Geometry check sheet. Reference: the model listing, model coordinates, mm. A direction names the side the tool comes from. Round coordinates to 2 decimals unless told otherwise and drop trailing zeros. Loops run counter-clockwise (first coordinate to the right, second up) from the corner with the lowest first, then second, coordinate; pieces in that order, holes last. Notation, with made-up numbers: (-29.5, 83.25) -> (-13.5, 83.25) arc R21 cw to (-13.5, 108.25) -> close; hole circle Ø4 at (75, -26). An arc over 180 degrees is marked (long way). Use a Markdown table: item, result. Add a question column.
Q1. Gauge pin test, flat ends, axial feed: P1, Ø5, axis at x = 7.5, z = 0, coming from the -Y side; P2, Ø1, axis at x = -1.5, z = 0, coming from the +Y side; P3, Ø2, axis at x = 7.5, z = 2, coming from the -Y side. Record the tip position at first contact, or that the pin passes through.
Q2. Set-up check for faces 4 (the face through (17.27, -0.9, 2.86)), 5 (the face through (22.152, 2, -1)), 6 (the face through (12.902, 3, 1)): record each of +Z, -Z, +X, -X, +Y, -Y from which the full face is reachable in a straight line by a thin tool's end or side.
Q3. Release check for a two-part mould opening along X. For faces 1 (the face through (16.21, -0.98, 3.11)), 2 (the face through (5, -3, 0)), 3 (the face through (-5.56, -0.71, -2.04)) record: released by +X, released by -X, zero draft, split by the parting line, or undercut.
Q4. Material ranges on L1, parallel to Y at x = 2.25, z = 0; L2, parallel to Z at x = 20.5, y = 1; L3, parallel to Z at x = 9, y = 0.75, recorded low to high.
Q5. Sectioned sample at A-A, the plane z = 0. Enter the section's corners in (x, y), then the cut area to 4 significant figures.
Q6. Sectioned sample at C-C, the plane x = 12.5. Enter the section's corners in (y, z), then the cut area to 3 significant figures.
Q7. Sectioned sample at B-B, the plane y = 0. Enter the section's corners in (x, z).
```python
from build123d import *

# Parameters (mm, degrees)
CUT_EXTRUDE1_DEPTH      = 10
CUT_EXTRUDE1_DEPTH_BACK = 10


with BuildPart() as part:
    # Sketch1 → Revolve1 (revolve)
    with BuildSketch(Plane.XY, mode=Mode.PRIVATE) as revolve1_sk:
        Polygon((22.151518872, 3), (17.651518872, 4.5), (17.651518872, 3), (16.901518872, 3), (12.901518872, 4.5), (12.901518872, 3), (-7.848481128, 3), (-7.848481128, 2), (22.151518872, 2), align=None)
    revolve(revolve1_sk.sketch.rotate(Axis((0, 0, 0), (1, 0, 0)), 90), axis=Axis((0, 0, 0), (1, 0, 0)))

    # Sketch2 → Cut-Extrude1 (cut, two sides: drawn at the far end of the back side and taken through both)
    with BuildSketch(Plane.XY.offset(-CUT_EXTRUDE1_DEPTH_BACK)):
        Polygon((-7.848481128, -3), (-1.848481128, 3), (-7.848481128, 3), align=None)
    extrude(amount=CUT_EXTRUDE1_DEPTH + CUT_EXTRUDE1_DEPTH_BACK, mode=Mode.SUBTRACT)


solid = part.part
```
Values:
| question | item | result |
|---|---|---|
| 1 | P1 | y = -3 |
| 1 | P2 | y = 3 |
| 1 | P3 | y = -2.83 |
| 2 | face 4 | none |
| 2 | face 5 | +Z, -Z, +X, +Y, -Y |
| 2 | face 6 | -X |
| 3 | face 1 | undercut |
| 3 | face 2 | zero draft |
| 3 | face 3 | released by -X |
| 4 | L1 | -3 to -2, 2 to 3 |
| 4 | L2 | -3.41 to -1.73, 1.73 to 3.41 |
| 4 | L3 | -2.9 to -1.85, 1.85 to 2.9 |
| 5 | outline | (-7.85, -3) -> (12.9, -3) -> (12.9, -4.5) -> (16.9, -3) -> (17.65, -3) -> (17.65, -4.5) -> (22.15, -3) -> (22.15, -2) -> (-6.85, -2) -> close; (-2.85, 2) -> (22.15, 2) -> (22.15, 3) -> (17.65, 4.5) -> (17.65, 3) -> (16.9, 3) -> (12.9, 4.5) -> (12.9, 3) -> (-1.85, 3) -> close |
| 5 | area | 66.75 mm^2 |
| 6 | outline | circle Ø6 at (0, 0); hole circle Ø4 at (0, 0) |
| 6 | area | 15.7 mm^2 |
| 7 | outline | (-4.85, -3) -> (12.9, -3) -> (12.9, -4.5) -> (16.9, -3) -> (17.65, -3) -> (17.65, -4.5) -> (22.15, -3) -> (22.15, -2) -> (-4.85, -2) -> close; (-4.85, 2) -> (22.15, 2) -> (22.15, 3) -> (17.65, 4.5) -> (17.65, 3) -> (16.9, 3) -> (12.9, 4.5) -> (12.9, 3) -> (-4.85, 3) -> close |
